```python
from build123d import *

# Parameters (mm, degrees)
BOSS_EXTRUDE1_DEPTH = 8.5
SHELL1_T            = -1.5
SKETCH3_W           = 14
SKETCH3_H           = 8.5
BOSS_EXTRUDE2_DEPTH = 1.5
CUT_EXTRUDE1_DEPTH  = 0.5
BOSS_EXTRUDE4_DEPTH = 1
FILLET2_R           = 1
SKETCH6_W           = 5.5
SKETCH6_H           = 2.6
BOSS_EXTRUDE5_DEPTH = 2
FILLET3_R           = 0.5
FILLET4_R           = 1


with BuildPart() as part:
    # Sketch1 → Boss-Extrude1 (new body)
    with BuildSketch(Plane.XY):
        Polygon((0, 0), (-6.5, 0), (-6.5, -10.5), (7.5, -10.5), (7.5, -8.3), (10.3, -8.3), (10.3, 0.1), (5.5, 0.1), (5.5, 5), (0, 5), align=None)
    extrude(amount=BOSS_EXTRUDE1_DEPTH)

    # Shell1
    shell1_openings = [part.faces().sort_by_distance(p)[0] for p in [
        (2.75, 5, 4.25),
        (5.5, 2.55, 4.25),
        (7.9, 0.1, 4.25),
        (0.5, -10.5, 4.25),
        (-3.25, 0, 4.25),
        (0, 2.5, 4.25),
    ]]
    offset(amount=SHELL1_T, openings=shell1_openings, kind=Kind.INTERSECTION)

    # Sketch3 → Boss-Extrude2 (add)
    with BuildSketch(Plane.XZ.offset(10.5)):
        with Locations((0.5, 4.25)):
            Rectangle(SKETCH3_W, SKETCH3_H)
    extrude(amount=-BOSS_EXTRUDE2_DEPTH)

    # Sketch4 → Cut-Extrude1 (cut)
    with BuildSketch(Plane.XZ.offset(10.5)):
        with BuildLine():
            Line((-3, 3.75), (-4.058316713, 1.916941682))
            ThreePointArc((-4.058316713, 1.916941682), (-3.875304011, 1.23392898), (-3.192291309, 1.416941682))
            Line((-3.192291309, 1.416941682), (-1.845299462, 3.75))
            Line((-1.845299462, 3.75), (-0.464100143, 3.75))
            Line((-0.464100143, 3.75), (-1.522416856, 1.916941682))
            ThreePointArc((-1.522416856, 1.916941682), (-1.339404154, 1.23392898), (-0.656391453, 1.416941682))
            Line((-0.656391453, 1.416941682), (0.690600395, 3.75))
            Line((0.690600395, 3.75), (2.071799714, 3.75))
            Line((2.071799714, 3.75), (1.013483001, 1.916941682))
            ThreePointArc((1.013483001, 1.916941682), (1.196495702, 1.23392898), (1.879508404, 1.416941682))
            Line((1.879508404, 1.416941682), (3.226500252, 3.75))
            Line((3.226500252, 3.75), (4.607699571, 3.75))
            Line((4.607699571, 3.75), (3.549382857, 1.916941682))
            ThreePointArc((3.549382857, 1.916941682), (3.732395559, 1.23392898), (4.415408261, 1.416941682))
            Line((4.415408261, 1.416941682), (5.762400109, 3.75))
            Line((5.762400109, 3.75), (5.90585335, 3.998468302))
            ThreePointArc((5.90585335, 3.998468302), (5.972840648, 4.248468302), (5.90585335, 4.498468302))
            Line((5.90585335, 4.498468302), (5.762400109, 4.746936604))
            Line((5.762400109, 4.746936604), (4.415408261, 7.079994922))
            ThreePointArc((4.415408261, 7.079994922), (3.732395559, 7.263007624), (3.549382857, 6.579994922))
            Line((3.549382857, 6.579994922), (4.607699571, 4.746936604))
            Line((4.607699571, 4.746936604), (3.226500252, 4.746936604))
            Line((3.226500252, 4.746936604), (1.879508404, 7.079994922))
            ThreePointArc((1.879508404, 7.079994922), (1.196495702, 7.263007624), (1.013483001, 6.579994922))
            Line((1.013483001, 6.579994922), (2.071799714, 4.746936604))
            Line((2.071799714, 4.746936604), (0.690600395, 4.746936604))
            Line((0.690600395, 4.746936604), (-0.656391453, 7.079994922))
            ThreePointArc((-0.656391453, 7.079994922), (-1.339404154, 7.263007624), (-1.522416856, 6.579994922))
            Line((-1.522416856, 6.579994922), (-0.464100143, 4.746936604))
            Line((-0.464100143, 4.746936604), (-1.845299462, 4.746936604))
            Line((-1.845299462, 4.746936604), (-3.192291309, 7.079994922))
            ThreePointArc((-3.192291309, 7.079994922), (-3.875304011, 7.263007624), (-4.058316713, 6.579994922))
            Line((-4.058316713, 6.579994922), (-3, 4.746936604))
            Line((-3, 4.746936604), (-2.856546759, 4.498468302))
            ThreePointArc((-2.856546759, 4.498468302), (-2.789559461, 4.248468302), (-2.856546759, 3.998468302))
            Line((-2.856546759, 3.998468302), (-3, 3.75))
        make_face()
    extrude(amount=-CUT_EXTRUDE1_DEPTH, mode=Mode.SUBTRACT)

    # Sketch5 → Boss-Extrude4 (add)
    with BuildSketch(Plane(origin=(0, 0.1, 0), x_dir=(1, 0, 0), z_dir=(0, 1, 0))):
        Polygon((10.3, 0.5), (8.3, 0.5), (8.3, 0), (10.3, 0), (10.3, -2), (10.8, -2), (10.8, 0.5), align=None)
        Polygon((10.8, -6.5), (10.3, -6.5), (10.3, -8.5), (8.3, -8.5), (8.3, -9), (10.3, -9), (10.8, -9), align=None)
    extrude(amount=-BOSS_EXTRUDE4_DEPTH)

    # Fillet2
    # the kernel refuses this fillet: 1 mm, written as the material it takes off along each edge
    with BuildSketch(Plane(origin=(8.3, 2.265063509, -0.5), x_dir=(0, 0, 1), z_dir=(0, -1, 0)), Plane(origin=(10.8, 2.265063509, 6.5), x_dir=(-1, 0, 0), z_dir=(0, -1, 0))) as fillet2_piece_1:
        with BuildLine():
            CenterArc((1, -0.866025404), FILLET2_R, 120, 60)
            Line((0, -0.866025404), (-0.02, -0.866025404))
            Line((-0.02, -0.866025404), (-0.02, 0))
            Line((-0.02, 0), (0, 0.02))
            ThreePointArc((0, 0.02), (0.25, 0.02), (0.49, 0.017320508))
            Line((0.49, 0.017320508), (0.5, 0))
        make_face()
    extrude(amount=5.330127019, mode=Mode.SUBTRACT)
    with BuildSketch(Plane(origin=(10.8, 2.265063509, 2), x_dir=(-1, 0, 0), z_dir=(0, -1, 0)), Plane(origin=(8.3, 2.265063509, 9), x_dir=(0, 0, -1), z_dir=(0, -1, 0))) as fillet2_piece_2:
        with BuildLine():
            CenterArc((1, 0.866025404), FILLET2_R, 180, 60)
            Line((0, 0.866025404), (-0.02, 0.866025404))
            Line((-0.02, 0.866025404), (-0.02, 0))
            Line((-0.02, 0), (0, -0.02))
            ThreePointArc((0, -0.02), (0.25, -0.02), (0.49, -0.017320508))
            Line((0.49, -0.017320508), (0.5, 0))
        make_face()
    extrude(amount=5.330127019, mode=Mode.SUBTRACT)
    with BuildSketch(Plane(origin=(10.8, 2.6, -0.5), x_dir=(-1, 0, 0), z_dir=(0, -1, 0))) as fillet2_piece_3:
        with BuildLine():
            CenterArc((FILLET2_R, -FILLET2_R), FILLET2_R, 90, 90)
            Line((0, -FILLET2_R), (-FILLET2_R * 0.02, -FILLET2_R))
            Line((-FILLET2_R * 0.02, -FILLET2_R), (-FILLET2_R * 0.02, FILLET2_R * 0.02))
            Line((-FILLET2_R * 0.02, FILLET2_R * 0.02), (FILLET2_R, FILLET2_R * 0.02))
            Line((FILLET2_R, FILLET2_R * 0.02), (FILLET2_R, 0))
        make_face()
    extrude(amount=6, mode=Mode.SUBTRACT)
    with BuildSketch(Plane(origin=(10.8, 2.6, 9), x_dir=(-1, 0, 0), z_dir=(0, -1, 0))) as fillet2_piece_4:
        with BuildLine():
            CenterArc((FILLET2_R, FILLET2_R), FILLET2_R, 180, 90)
            Line((0, FILLET2_R), (-FILLET2_R * 0.02, FILLET2_R))
            Line((-FILLET2_R * 0.02, FILLET2_R), (-FILLET2_R * 0.02, -FILLET2_R * 0.02))
            Line((-FILLET2_R * 0.02, -FILLET2_R * 0.02), (FILLET2_R, -FILLET2_R * 0.02))
            Line((FILLET2_R, -FILLET2_R * 0.02), (FILLET2_R, 0))
        make_face()
    extrude(amount=6, mode=Mode.SUBTRACT)

    # Sketch6 → Boss-Extrude5 (add)
    with BuildSketch(Plane(origin=(0, 5, 0), x_dir=(1, 0, 0), z_dir=(0, 1, 0))):
        with Locations((2.75, -8.3)):
            Rectangle(SKETCH6_W, SKETCH6_H)
        with Locations((2.75, -0.2)):
            Rectangle(SKETCH6_W, SKETCH6_H)
    extrude(amount=-BOSS_EXTRUDE5_DEPTH)

    # Fillet3
    fillet3_edges = [part.edges().sort_by_distance(p)[0] for p in [
        (10.3, -4.6, 0),
        (8.9, -8.3, 0),
        (7.5, -9.4, 0),
        (0.5, -10.5, 0),
        (-6.5, -5.25, 8.5),
        (-6.5, -5.25, 0),
        (0.5, -10.5, 8.5),
        (10.3, -8.3, 4.25),
        (7.5, -8.3, 4.25),
        (7.5, -10.5, 4.25),
        (-6.5, -10.5, 4.25),
        (7.5, -9.4, 8.5),
        (8.9, -8.3, 8.5),
        (10.3, -4.6, 8.5),
    ]]
    fillet(fillet3_edges, radius=FILLET3_R)

    # Fillet4
    fillet4_edges = [part.edges().sort_by_distance(p)[0] for p in [
        (0, 2.5, 1.5),
        (5.5, 2.55, 1.5),
        (0, 2.5, 7),
        (5.5, 2.55, 7),
    ]]
    fillet(fillet4_edges, radius=FILLET4_R)


solid = part.part
```
Model file for the job. Use its own axes, mm. A direction names the side the tool comes from. Round coordinates to 2 decimals unless told otherwise and drop trailing zeros. Order: outer loops, then holes, each group sorted by start corner. A loop starts at its lowest first (then second) coordinate and runs counter-clockwise, first axis right, second up. Notation, with made-up numbers: (1, 68.5) -> (24, 68.5) arc R18 ccw to (24, 75.5) -> close; hole circle Ø3 at (-33, 75). An arc over 180 degrees is marked (long way). Use one line per item in the form item = value.
Item 1: Drill centre lines: line 1 (Z direction, x = 4.5, y = 0); line 2 (Y direction, x = 1.75, z = 6); line 3 (Z direction, x = 0.5, y = 3.25). Where is each one in solid material? Low to high.
Returned:
line_1 = 0 to 1.5, 7 to 8.5
line_2 = -10 to -9
line_3 = -1.1 to 1.37, 7.13 to 9.6
Item 2: Cut at B-B, the plane y = -2.5. Write the cut outline in (x, z), and give its area (3 significant figures).
Returned:
outline = (-6.5, 0.5) arc R0.5 ccw to (-6, 0) -> (9.8, 0) arc R0.5 ccw to (10.3, 0.5) -> (10.3, 8) arc R0.5 ccw to (9.8, 8.5) -> (-6, 8.5) arc R0.5 ccw to (-6.5, 8) -> close; hole (-5, 1.5) -> (8.8, 1.5) -> (8.8, 7) -> (-5, 7) -> close
area = 66.7 mm^2
Item 3: Flat gauge pins, fed straight in: pin 1 Ø6 at (x, z) = (-2.5, 6) entering from +Y; pin 2 Ø0.5 at (x, z) = (8.5, 2.5) entering from -Y; pin 3 Ø1 at (x, z) = (8.5, 8.5) entering from +Y; pin 4 Ø1.8 at (x, z) = (0.5, 5) entering from -Y. Where does each tip first touch, or does it go through?
Returned:
pin_1 = 0
pin_2 = -8.3
pin_3 = 0.1
pin_4 = -10.5
Item 4: Pull direction X, two halves, no side cores. Call faces 1 (the face through (4.07, -10.25, 5.68)), 2 (the face through (9, 0.1, 5)), 3 (the face through (10.515, -0.393, 8.699)), 4 (the face through (4.09, -10.25, 2.85)): released by +X, released by -X, zero draft, split by the parting line, or undercut.
Returned:
face_1 = undercut
face_2 = zero draft
face_3 = released by +X
face_4 = undercut
Item 5: Tool access for faces 5 (the face through (9, -8.3, 4)), 6 (the face through (6, -8, 4)), 7 (the face through (0.301, 2.465, 7.285)), 8 (the face through (-2.528, -10.254, 2.567)): list every direction of +Z, -Z, +X, -X, +Y, -Y with a clear straight run to the whole face (end or side of a thin tool).
Returned:
face_5 = +Z, -Z, +X, -Y
face_6 = +Y
face_7 = -X, +Y
face_8 = -Y
Item 6: Cut at A-A, the plane y = 0.75. Write the cut outline in (x, z).
Returned:
outline = (0, 0) -> (5.5, 0) -> (5.5, 0.5) arc R1 ccw to (4.5, 1.5) -> (1, 1.5) arc R1 ccw to (0, 0.5) -> close; (0, 8) arc R1 ccw to (1, 7) -> (4.5, 7) arc R1 ccw to (5.5, 8) -> (5.5, 8.5) -> (0, 8.5) -> close
Item 7: Cut at D-D, the plane x = 2.5. Write the cut outline in (y, z), and give its area (3 significant figures).
Returned:
outline = (-10.5, 0.5) arc R0.5 ccw to (-10, 0) -> (3, 0) -> (3, -1.1) -> (5, -1.1) -> (5, 1.5) -> (-9, 1.5) -> (-9, 7) -> (5, 7) -> (5, 9.6) -> (3, 9.6) -> (3, 8.5) -> (-10, 8.5) arc R0.5 ccw to (-10.5, 8) -> (-10.5, 6.01) -> (-10, 6.01) -> (-10, 2.49) -> (-10.5, 2.49) -> close
area = 57.3 mm^2
